```python
from build123d import *

# Parameters (mm, degrees)
SKETCH_2_W      = 40
SKETCH_2_H      = 40
EXTRUDE_1_DEPTH = 21
SKETCH_3_R      = 15
EXTRUDE_2_DEPTH = 50
SKETCH_4_R      = 22.5
EXTRUDE_3_DEPTH = 6
CHAMFER_1_SIZE  = 5
FILLET_1_R      = 1


with BuildPart() as part:
    # 草图2 → 凸台-拉伸1 (new body)
    with BuildSketch(Plane(origin=(0, 0, 0), x_dir=(1, 0, 0), z_dir=(0, 1, 0))):
        Rectangle(SKETCH_2_W, SKETCH_2_H)
    extrude(amount=EXTRUDE_1_DEPTH)

    # 草图3 → 凸台-拉伸2 (add)
    with BuildSketch(Plane(origin=(0, 21, 0), x_dir=(1, 0, 0), z_dir=(0, 1, 0))):
        Circle(SKETCH_3_R)
    extrude(amount=EXTRUDE_2_DEPTH)

    # 草图4 → 凸台-拉伸3 (add)
    with BuildSketch(Plane(origin=(0, 71, 0), x_dir=(1, 0, 0), z_dir=(0, 1, 0))):
        Circle(SKETCH_4_R)
    extrude(amount=EXTRUDE_3_DEPTH)

    # 倒角1
    chamfer_1_edges = [part.edges().sort_by_distance(p)[0] for p in [
        (-15, 71, 0),
    ]]
    chamfer(chamfer_1_edges, length=CHAMFER_1_SIZE)

    # 圆角1
    fillet_1_edges = [part.edges().sort_by_distance(p)[0] for p in [
        (-15, 21, 0),
        (-22.5, 71, 0),
        (-22.5, 77, 0),
        (-20, 71, 0),
        (-15, 66, 0),
    ]]
    fillet(fillet_1_edges, radius=FILLET_1_R)


solid = part.part
```
The listing builds one solid part. Answer for the finished solid, in the listing's coordinates (mm). A direction names the side the tool comes from. Give positions to 0.01 mm unless a question says otherwise; leave off trailing zeros. Loops run counter-clockwise (first coordinate to the right, second up) from the corner with the lowest first, then second, coordinate; pieces in that order, holes last. Notation, with made-up numbers: M -27.5,-39 L -8.5,-39 A19 cw -8.5,-11 Z; hole C -34,-6 d5. An arc over 180 degrees is marked long. One line per item, written item: value.
1. For a pull along Y with two mould halves and no side action, classify faces 1 (the face through (0, 0, 0)), 2 (the face through (0, 10, 20)), 3 (the face through (0, 77, 0)), 4 (the face through (7.16, 66.51, 13.76)) as pulls with the +Y half, pulls with the -Y half, needs draft (parallel to the pull), parting line crosses it, or undercut.
Found:
face 1: pulls with the -Y half
face 2: needs draft
face 3: pulls with the +Y half
face 4: undercut
2. Each of these flat-tipped pins is pushed along its axis until it touches: P1, Ø23, axis at x = -5, y = 10.5, coming from the +Z side; P2, Ø12, axis at y = 47.5, z = -6, coming from the +X side; P3, Ø2, axis at y = 11, z = 1.5, coming from the -X side. Where does it stop, or does it pass through?
Found:
P1: z = 20
P2: x = 15
P3: x = -20
3. Section C-C on y = 16 is taken. Determine the outline of the cut face in (x, z), plus the area to 3 significant figures.
Found:
outline: M -20,-20 L 20,-20 L 20,20 L -20,20 Z
area: 1,600 mm^2
4. Section A-A on y = 68.5 is taken. Determine the outline of the cut face in (x, z).
Found:
outline: C 0,0 d35
5. Section B-B on y = 53.5 is taken. Determine the outline of the cut face in (x, z), plus the area to 3 significant figures.
Found:
outline: C 0,0 d30
area: 707 mm^2
6. Find the intervals of material crossed by probe 1 along Z at (x, y) = (-15, 6); probe 2 along Y at (x, z) = (17, 18), in increasing order.
Found:
probe 1: -20 to 20
probe 2: 0 to 21
7. For faces 5 (the face through (10.382, 73.972, 19.961)), 6 (the face through (13.856, 43.488, 5.745)), 7 (the face through (20, 10, 0)), 8 (the face through (-20, 10, 0)), determine the directions among +Z, -Z, +X, -X, +Y, -Y from which every point of the face is accessible in a straight line to the end or side of a thin tool.
Found:
face 5: +Y
face 6: none
face 7: +Z, -Z, +X, -Y
face 8: +Z, -Z, -X, -Y
